```python
from build123d import *

# Parameters (mm, degrees)
SKETCH_1_R                 = 1
EXTRUDE_1_DEPTH            = 2
M3X0_51_AT_2_COUNT         = 2
M3X0_51_AT_2_PITCH         = 9.998489886
HOLE_WIZARD_M31_AT_2_COUNT = 2
HOLE_WIZARD_M31_AT_2_PITCH = 9.998489886


with BuildPart() as part:
    # Эскиз1 → Бобышка-Вытянуть1 (new body)
    with BuildSketch(Plane.XY):
        Polygon((0, 15.5), (1.5, 17), (15.5, 17), (17, 15.5), (17, 1.5), (15.5, 0), (1.5, 0), (0, 1.5), align=None)
        with Locations((5, 5)):
            Circle(SKETCH_1_R, mode=Mode.SUBTRACT)
        with Locations((12.07, 5)):
            Circle(SKETCH_1_R, mode=Mode.SUBTRACT)
        with Locations((12.07, 12.07)):
            Circle(SKETCH_1_R, mode=Mode.SUBTRACT)
        with Locations((5, 12.07)):
            Circle(SKETCH_1_R, mode=Mode.SUBTRACT)
    extrude(amount=EXTRUDE_1_DEPTH)

    # Эскиз2 → Отверстие обработанное метчиком M3x0.51 (revolve, cut)
    with BuildSketch(Plane(origin=(12.07, 12.07, 2), x_dir=(0, -1, 0), z_dir=(1, 0, 0))):
        Polygon((0, 0), (0, 2), (1.6, 2), (1.25, 1.797927406), (1.25, 0.202072594), (1.6, 0), align=None)
    m3x0_51 = revolve(axis=Axis((12.07, 12.07, 8.35), (0, 0, -1)), mode=Mode.SUBTRACT)

    # Отверстие обработанное метчиком M3x0.51 at 2: Отверстие обработанное метчиком M3x0.51 ×2
    with Locations(*[Vector(-0.707106781, -0.707106781, 0) * (i * M3X0_51_AT_2_PITCH) for i in range(1, M3X0_51_AT_2_COUNT)]):
        add(m3x0_51, mode=Mode.SUBTRACT)

    # Эскиз4 → Цековка для винта с заклепочной головкой M31 (revolve, cut)
    with BuildSketch(Plane(origin=(5, 12.07, 2), x_dir=(0, -1, 0), z_dir=(1, 0, 0))):
        Polygon((0, 0), (0, 2), (1.85, 2), (1.8, 1.95), (1.8, 1.3), (3.75, 1.3), (3.75, 0.05), (3.8, 0), align=None)
    hole_wizard_m31 = revolve(axis=Axis((5, 12.07, 8.35), (0, 0, -1)), mode=Mode.SUBTRACT)

    # Цековка для винта с заклепочной головкой M31 at 2: Цековка для винта с заклепочной головкой M31 ×2
    with Locations(*[Vector(0.707106781, -0.707106781, 0) * (i * HOLE_WIZARD_M31_AT_2_PITCH) for i in range(1, HOLE_WIZARD_M31_AT_2_COUNT)]):
        add(hole_wizard_m31, mode=Mode.SUBTRACT)


solid = part.part
```
Could you check a few things on this model? Use its own coordinates, in mm. A direction names the side the tool comes from. Round coordinates to 2 decimals unless told otherwise and drop trailing zeros. Loops run counter-clockwise (first coordinate to the right, second up) from the corner with the lowest first, then second, coordinate; pieces in that order, holes last.
Q1. Thinking about a two-plate mould opening in Y: for faces 3 (the flat face through (0.8, 0.7, 1)), 4 (the cylindrical face through (14.352, 7.976, 1.334)), 5 (the flat face through (0.7, 16.2, 1)), which applies, pulls with the +Y half, pulls with the -Y half, needs draft (parallel to the pull), parting line crosses it, or undercut?
Q2. On a 3-axis mill with a long thin cutter (end or side, diameter ignored), from which of +Z, -Z, +X, -X, +Y, -Y can I reach the whole of each face in a straight line? I mean faces 1 (the cylindrical face through (6.436, 8.606, 1.334)), 2 (the flat face through (17, 9, 1)). Say none if no direction works.
Q3. I want a section at A-A (z = 1.2). Write out the boundary of the cut face in (x, y), and give its area (3 significant figures).
Q4. Please list where these lines run through material, in increasing order: L1, parallel to X at y = 5, z = 1.2; L2, parallel to X at y = 12.07, z = 1.65.
Q5. For P1, Ø4, axis at x = 6, y = 11.5, coming from the +Z side; P2, Ø7, axis at x = 12.07, y = 5, coming from the -Z side, each with a flat end and sliding along its axis, tell me the tip position at first contact or that it passes through.
Q6. I want a section at B-B (x = 12.07). Write out the boundary of the cut face in (y, z).
Answer below:
1. face 3: pulls with the -Y half
1. face 4: undercut
1. face 5: pulls with the +Y half
2. face 1: +Z
2. face 2: +Z, -Z, +X, +Y, -Y
3. outline: (0, 1.5) - (1.5, 0) - (15.5, 0) - (17, 1.5) - (17, 15.5) - (15.5, 17) - (1.5, 17) - (0, 15.5) - close; hole circle Ø7.5 at (5, 12.07); hole circle Ø2.5 at (5, 5); hole circle Ø7.5 at (12.07, 5); hole circle Ø2.5 at (12.07, 12.07)
3. area: 186 mm2
4. L1: x = 0 to 3.75, 6.25 to 8.32, 15.82 to 17
4. L2: x = 0 to 1.25, 8.75 to 10.82, 13.32 to 17
5. P1: stops at z = 0.7
5. P2: stops at z = 0
6. outline: (0, 0) - (3.15, 0) - (3.2, 0.05) - (3.2, 0.7) - (1.25, 0.7) - (1.25, 1.95) - (1.2, 2) - (0, 2) - close; (6.8, 0.05) - (6.85, 0) - (10.47, 0) - (10.82, 0.2) - (10.82, 1.8) - (10.47, 2) - (8.8, 2) - (8.75, 1.95) - (8.75, 0.7) - (6.8, 0.7) - close; (13.32, 0.2) - (13.67, 0) - (17, 0) - (17, 2) - (13.67, 2) - (13.32, 1.8) - close
